Can you work these out from the model? Positions are in its coordinate system, mm. Give positions to 0.01 mm unless a question says otherwise; leave off trailing zeros. Answer as a JSON object with one key per item and string values.
```python
from build123d import *

# Parameters (mm, degrees)
F0_R      = 0.254
F1_DEPTH  = 27.94
F4_R      = 0.254
F5_DEPTH  = 27.94
F7_R      = 0.254
F8_DEPTH  = 27.94
F11_R     = 0.254
F12_DEPTH = 27.94
F14_R     = 0.254
F15_DEPTH = 27.94
F18_R     = 0.254
F19_DEPTH = 28.0416
F21_R     = 0.254
F22_DEPTH = 28.0416
F24_R     = 0.254
F25_DEPTH = 28.0416
F27_R     = 0.254
F28_DEPTH = 28.0416


with BuildPart() as f1:
    # F0 (on Front) → F1 (new body)
    with BuildSketch(Plane.XZ):
        Circle(F0_R)
    extrude(amount=F1_DEPTH)

    # F4 (on line) → F5 (join)
    with BuildSketch(Plane(origin=(0, 0, 0), x_dir=(-0.9961946981, 0.0871557427, 0), z_dir=(0.0871557427, 0.9961946981, 0))):
        Circle(F4_R)
    extrude(amount=-F5_DEPTH)

    # F7 (on line) → F8 (join)
    with BuildSketch(Plane(origin=(0, 0, 0), x_dir=(0.9961946981, 0.0871557427, 0), z_dir=(0.0871557427, -0.9961946981, 0))):
        Circle(F7_R)
    extrude(amount=F8_DEPTH)

    # F11 (on line) → F12 (join)
    with BuildSketch(Plane(origin=(0, 0, 0), x_dir=(-1, 0, 0), z_dir=(0, 0.9961946981, 0.0871557427))):
        Circle(F11_R)
    extrude(amount=-F12_DEPTH)

    # F14 (on line) → F15 (join)
    with BuildSketch(Plane(origin=(0, 0, 0), x_dir=(1, 0, 0), z_dir=(0, -0.9961946981, 0.0871557427))):
        Circle(F14_R)
    extrude(amount=F15_DEPTH)

    # F18 (on line) → F19 (join)
    with BuildSketch(Plane(origin=(0, 0, 0), x_dir=(-0.9967911096, -0.0797882397, -0.0064281109), z_dir=(-0.0800467601, 0.9935718557, 0.0800467601))):
        Circle(F18_R)
    extrude(amount=-F19_DEPTH)

    # F21 (on line) → F22 (join)
    with BuildSketch(Plane(origin=(0, 0, 0), x_dir=(0.9967911096, -0.0797882397, 0.0064281109), z_dir=(-0.0800467601, -0.9935718557, 0.0800467601))):
        Circle(F21_R)
    extrude(amount=F22_DEPTH)

    # F24 (on line) → F25 (join)
    with BuildSketch(Plane(origin=(0, 0, 0), x_dir=(-0.9967911096, -0.0797882397, 0.0064281109), z_dir=(-0.0800467601, 0.9935718557, -0.0800467601))):
        Circle(F24_R)
    extrude(amount=-F25_DEPTH)

    # F27 (on line) → F28 (join)
    with BuildSketch(Plane(origin=(0, 0, 0), x_dir=(0.9967911096, -0.0797882397, -0.0064281109), z_dir=(-0.0800467601, -0.9935718557, -0.0800467601))):
        Circle(F27_R)
    extrude(amount=F28_DEPTH)


solid = f1.part
```
1) I'm going to push flat-ended pins straight in: P1, Ø1, axis at y = -20.5, z = 1.5, coming from the +X side; P2, Ø2, axis at x = 2, z = -2, coming from the -Y side; P3, Ø1.5, axis at x = 0, y = -11.5, coming from the -Z side. Where does each tip first touch, or does it pass through?
Check sheet entries:
{"P1": "x = 1.94", "P2": "y = -27.89", "P3": "z = -1.33"}
2) If we mould it in two halves opening along Z, with no side actions, what happens to faces 1 (the cylindrical face through (-0.033, -16.793, 1.722)), 2 (the cylindrical face through (1.54, -16.8, 1.53))? For each: released by +Z, released by -Z, zero draft, split by the parting line, or undercut.
Check sheet entries:
{"face 1": "undercut", "face 2": "undercut"}
3) I need wall thicknesses on L1, parallel to X at y = -20.5, z = 0.15; L2, parallel to X at y = -16, z = 0.05; L3, parallel to X at y = -24.5, z = 2.3. Which ranges of each line are inside material? Lowest first, please.
Check sheet entries:
{"L1": "-2 to -1.59, -0.2 to 0.2, 1.59 to 2", "L2": "-1.65 to -1.15, -0.25 to 0.25, 1.15 to 1.65", "L3": "-0.2 to 0.2"}
4) Imagine slicing it at A-A on y = -14.5. Give the number of separate pieces and of enclosed holes in the cut face, and give its area (3 significant figures).
Check sheet entries:
{"separate pieces": "9", "enclosed holes": "0", "area": "1.83 mm2"}
